Read the model definition and answer for the solid it produces. Units are mm, in the model's axes. Coordinates: 2 decimals unless noted, no trailing zeros. Write each loop counter-clockwise with the first axis right and the second up, starting at its lowest first coordinate (ties: lowest second). Pieces come first, ordered by that corner, then holes.
Item 1: Each of these flat-tipped pins is pushed along its axis until it touches: P1, Ø3.5, axis at y = -12.7, z = 187.325, coming from the +X side; P2, Ø7, axis at y = -12.7, z = -187.325, coming from the -X side. Where does it stop, or does it pass through?
Item 2: Straight lines are drawn through the part: probe 1 along Z at (x, y) = (5.4, -12.7); probe 2 along Z at (x, y) = (2.75, -33); probe 3 along Y at (x, z) = (1, 186.5). For each, find the intervals that lie inside material, in ascending order.
Item 3: Section C-C (z = 132) is taken. Give the vertices of the cut face in (x, y).
Item 4: Section A-A (y = -185) is taken. Give the vertices of the cut face in (x, z), then the cut area to 3 significant figures.
Item 5: Section B-B (x = 4.75) is taken. Give the vertices of the cut face in (y, z) (3 decimals).
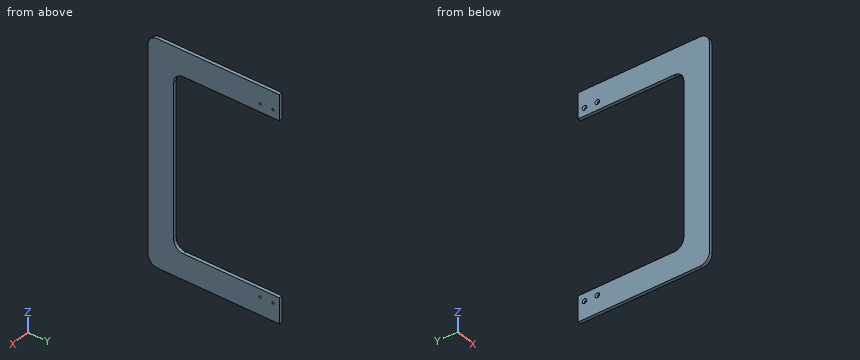
from build123d import *

# Parameters (mm, degrees)
BOSS_EXTRUDE2_DEPTH                               = 6.35
CSK_FOR_8_FLAT_HEAD_SOCKET_CAP_SCREW1_D           = 4.3053
CSK_FOR_8_FLAT_HEAD_SOCKET_CAP_SCREW1_CSINK_D     = 9.1186
CSK_FOR_8_FLAT_HEAD_SOCKET_CAP_SCREW1_CSINK_ANGLE = 82


with BuildPart() as part:
    # Sketch1 → Boss-Extrude2 (new body)
    with BuildSketch(Plane(origin=(0, 0, 0), x_dir=(0, 0, -1), z_dir=(1, 0, 0))):
        with BuildLine():
            Line((-222.25, 0), (-171.45, 0))
            Line((-171.45, 0), (-171.45, -190.5))
            ThreePointArc((-171.45, -190.5), (-165.870384182, -203.970384182), (-152.4, -209.55))
            Line((-152.4, -209.55), (152.4, -209.55))
            ThreePointArc((152.4, -209.55), (165.870384182, -203.970384182), (171.45, -190.5))
            Line((171.45, -190.5), (171.45, 0))
            Line((171.45, 0), (222.25, 0))
            Line((222.25, 0), (222.25, -241.3))
            ThreePointArc((222.25, -241.3), (216.670384182, -254.770384182), (203.2, -260.35))
            Line((203.2, -260.35), (-203.2, -260.35))
            ThreePointArc((-203.2, -260.35), (-216.670384182, -254.770384182), (-222.25, -241.3))
            Line((-222.25, -241.3), (-222.25, 0))
        make_face()
    extrude(amount=BOSS_EXTRUDE2_DEPTH)

    # CSK for #8 Flat Head Socket Cap Screw1 (through all)
    with Locations(Plane.ZY):
        with Locations((-187.325, -12.7), (-187.325, -38.1)):
            csk_for_8_flat_head_socket_cap_screw1 = CounterSinkHole(CSK_FOR_8_FLAT_HEAD_SOCKET_CAP_SCREW1_D / 2, CSK_FOR_8_FLAT_HEAD_SOCKET_CAP_SCREW1_CSINK_D / 2, counter_sink_angle=CSK_FOR_8_FLAT_HEAD_SOCKET_CAP_SCREW1_CSINK_ANGLE)

    # Mirror1: CSK for #8 Flat Head Socket Cap Screw1 across plane
    add(csk_for_8_flat_head_socket_cap_screw1.mirror(Plane.XY), mode=Mode.SUBTRACT)


solid = part.part
Established:
1. P1: passes through
1. P2: stops at x = 1.22
2. probe 1: z = -222.25 to -189.48, -185.17 to -171.45, 171.45 to 185.17, 189.48 to 222.25
2. probe 2: z = -222.25 to -171.45, 171.45 to 222.25
2. probe 3: y = -260.35 to -41.7, -34.5 to -16.3, -9.1 to 0
3. outline: (0, -260.35) - (6.35, -260.35) - (6.35, -209.55) - (0, -209.55) - close
4. outline: (0, -222.25) - (6.35, -222.25) - (6.35, -171.45) - (0, -171.45) - close; (0, 171.45) - (6.35, 171.45) - (6.35, 222.25) - (0, 222.25) - close
4. area: 645 mm2
5. outline: (-260.35, -203.2) arc R19.05 ccw to (-241.3, -222.25) - (0, -222.25) - (0, -171.45) - (-190.5, -171.45) arc R19.05 cw to (-209.55, -152.4) - (-209.55, 152.4) arc R19.05 cw to (-190.5, 171.45) - (0, 171.45) - (0, 222.25) - (-241.3, 222.25) arc R19.05 ccw to (-260.35, 203.2) - close; hole circle Ø4.305 at (-38.1, -187.325); hole circle Ø4.305 at (-38.1, 187.325); hole circle Ø4.305 at (-12.7, -187.325); hole circle Ø4.305 at (-12.7, 187.325)
